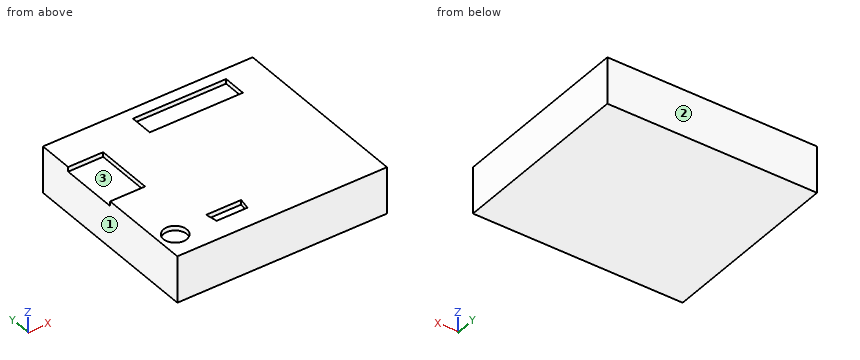
```python
from build123d import *

# Parameters (mm, degrees)
ESQUISSE1_W             = 90
ESQUISSE1_H             = 80
BOSS_EXTRU_1_DEPTH      = 20
ESQUISSE2_W             = 40
ESQUISSE2_H             = 10
ENL_V_MAT_EXTRU_1_DEPTH = 2
ENL_V_MAT_EXTRU_2_DEPTH = 2
ESQUISSE4_R             = 5
ENL_V_MAT_EXTRU_3_DEPTH = 2
ESQUISSE5_W             = 15
ESQUISSE5_H             = 25
ENL_V_MAT_EXTRU_4_DEPTH = 2


with BuildPart() as part:
    # Esquisse1 → Boss.-Extru.1 (new body)
    with BuildSketch(Plane.XY):
        Rectangle(ESQUISSE1_W, ESQUISSE1_H)
    extrude(amount=BOSS_EXTRU_1_DEPTH)

    # Esquisse2 → Enlèv. mat.-Extru.1 (cut)
    with BuildSketch(Plane.XY.offset(20)):
        with Locations((10, 30)):
            Rectangle(ESQUISSE2_W, ESQUISSE2_H)
    extrude(amount=-ENL_V_MAT_EXTRU_1_DEPTH, mode=Mode.SUBTRACT)

    # Esquisse3 → Enlèv. mat.-Extru.2 (cut)
    with BuildSketch(Plane.XY.offset(20)):
        Polygon((-8.381634904, -31), (-21.618365096, -31), (-22.5, -26), (-7.5, -26), align=None)
    extrude(amount=-ENL_V_MAT_EXTRU_2_DEPTH, mode=Mode.SUBTRACT)

    # Esquisse4 → Enlèv. mat.-Extru.3 (cut)
    with BuildSketch(Plane.XY.offset(20)):
        with Locations((-38, -29)):
            Circle(ESQUISSE4_R)
    extrude(amount=-ENL_V_MAT_EXTRU_3_DEPTH, mode=Mode.SUBTRACT)

    # Esquisse5 → Enlèv. mat.-Extru.4 (cut)
    with BuildSketch(Plane.XY.offset(20)):
        with Locations((-37.5, 12.5)):
            Rectangle(ESQUISSE5_W, ESQUISSE5_H)
    extrude(amount=-ENL_V_MAT_EXTRU_4_DEPTH, mode=Mode.SUBTRACT)


solid = part.part
```
Here's how the part is built. I have some questions about the finished solid (model axes, mm). Face numbers are marked on the shaded views. Coordinates: 2 decimals unless noted, no trailing zeros. Write each loop counter-clockwise with the first axis right and the second up, starting at its lowest first coordinate (ties: lowest second). Pieces come first, ordered by that corner, then holes. Notation, with made-up numbers: (75.25, 79.25) -> (84.25, 79.25) arc R17 ccw to (84.25, 110.25) -> close; hole circle Ø9 at (22, -33). An arc over 180 degrees is marked (long way). Use a Markdown table: item, result. Add a question column.
(1) If we section it at B-B, the plane y = -28: Write out the boundary of the cut face in (x, z).
(2) We'd pull the mould along Y, two halves only. Please class the marked faces 1, 2 and 3: +Y half, -Y half, draft (parallel to the pull), parting line (faces both ways), or undercut.
(3) If we section it at A-A, the plane x = -38: Write out the boundary of the cut face in (y, z), and give its area (3 significant figures).
(4) I'm going to push flat-ended pins straight in: P1, Ø5, axis at x = 32.5, y = 0.5, coming from the -Z side; P2, Ø4, axis at x = 25.5, y = 29.5, coming from the +Z side; P3, Ø0.6, axis at y = 12.5, z = 19, coming from the -X side. Where does each tip first touch, or does it pass through?
(5) Please list where these lines run through material, in increasing order: line 1 (Y direction, x = -38, z = 19.2); line 2 (Z direction, x = 15, y = 33).
Outcome:
| question | item | result |
|---|---|---|
| 1 | outline | (-45, 0) -> (45, 0) -> (45, 20) -> (-7.85, 20) -> (-7.85, 18) -> (-22.15, 18) -> (-22.15, 20) -> (-33.1, 20) -> (-33.1, 18) -> (-42.9, 18) -> (-42.9, 20) -> (-45, 20) -> close |
| 2 | face 1 | draft |
| 2 | face 2 | +Y half |
| 2 | face 3 | undercut |
| 3 | outline | (-40, 0) -> (40, 0) -> (40, 20) -> (25, 20) -> (25, 18) -> (0, 18) -> (0, 20) -> (-24, 20) -> (-24, 18) -> (-34, 18) -> (-34, 20) -> (-40, 20) -> close |
| 3 | area | 1,530 mm^2 |
| 4 | P1 | stops at z = 0 |
| 4 | P2 | stops at z = 18 |
| 4 | P3 | stops at x = -30 |
| 5 | line 1 | y = -40 to -34, -24 to 0, 25 to 40 |
| 5 | line 2 | z = 0 to 18 |
